Job drawing, mm, ordinate dimensions from the low corner. One solid piece. A direction names the side the tool comes from. Give positions to 0.01 mm unless a question says otherwise; leave off trailing zeros. Loops run counter-clockwise (first coordinate to the right, second up) from the corner with the lowest first, then second, coordinate; pieces in that order, holes last. Notation, with made-up numbers: M -29,39.25 L -3,39.25 A32 ccw -3,76.25 Z; hole C 64,17.25 d11. An arc over 180 degrees is marked long. Put each result on its own line as item: value.
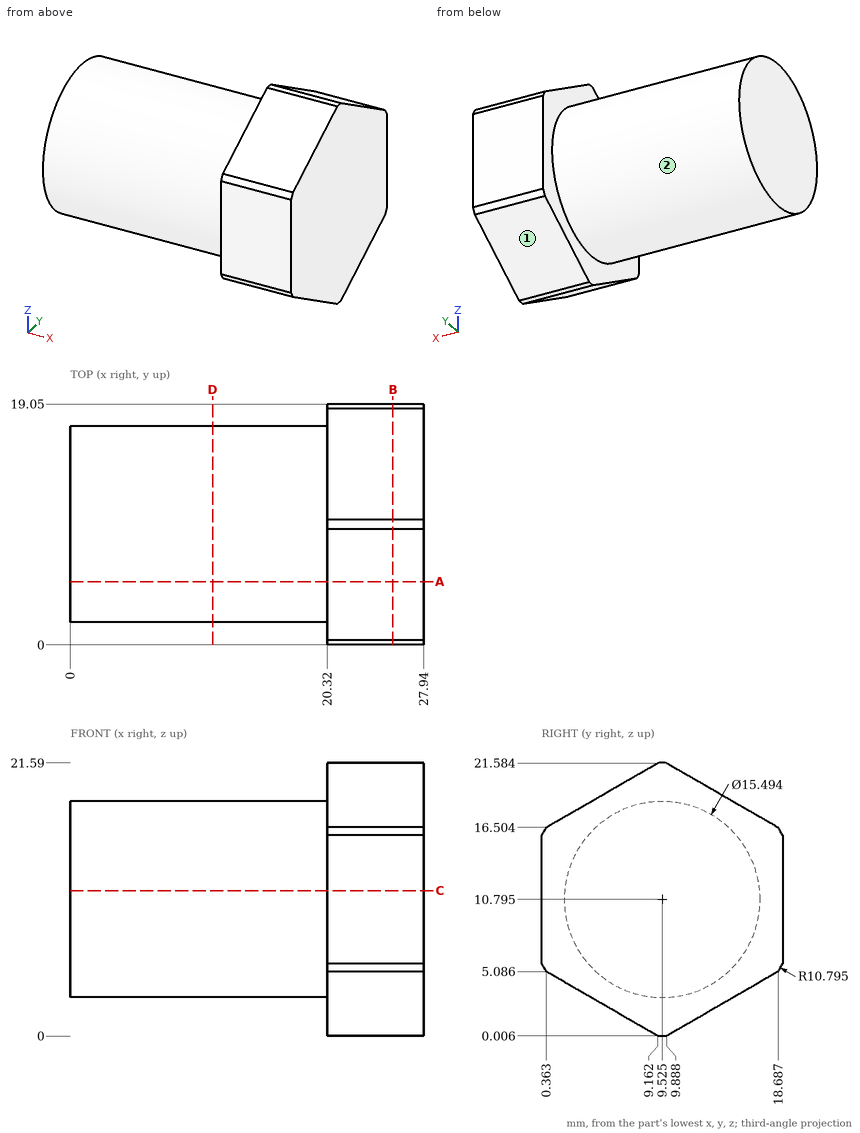
Q1. Slice it at A-A (y = 5). List the corners of the cut face in (x, z).
Here are the results:
outline: M 0,4.51 L 20.32,4.51 L 20.32,2.41 L 27.94,2.41 L 27.94,19.18 L 20.32,19.18 L 20.32,17.08 L 0,17.08 Z
Q2. Drop flat-ended pins along their axis: pin 1 Ø3 at (x, y) = (9, 16) entering from -Z; pin 2 Ø4 at (x, y) = (19.5, 17) entering from -Z; pin 3 Ø6 at (x, z) = (9.5, 5) entering from +Y. Give the stop position or say it passes through.
Here are the results:
pin 1: z = 4.86
pin 2: z = 3.06
pin 3: y = 16.75
Q3. Slice it at D-D (x = 11.25). List the corners of the cut face in (y, z) (3 decimals).
Here are the results:
outline: C 9.525,10.795 d15.494
Q4. Probe line 1 (X direction, y = 2, z = 7.5); line 2 (Z direction, x = 19.75, y = 9.75); line 3 (Z direction, x = 25.5, y = 3.5) (3 decimals). List the from-to ranges inside material, lowest first. Write a range as from..to.
Here are the results:
line 1: 20.32..27.94
line 2: 3.05..18.54
line 3: 3.275..18.315
Q5. Slice it at B-B (x = 25.5). List the corners of the cut face in (y, z) (3 decimals), and give its area (3 significant figures).
Here are the results:
outline: M 0,5.715 A10.795 ccw 0.363,5.086 L 9.162,0.006 A10.795 ccw 9.888,0.006 L 18.687,5.086 A10.795 ccw 19.05,5.715 L 19.05,15.875 A10.795 ccw 18.687,16.504 L 9.888,21.584 A10.795 ccw 9.162,21.584 L 0.363,16.504 A10.795 ccw 0,15.875 Z
area: 314 mm²
Q6. Tool access for the marked faces 1 and 2: list every direction of +Z, -Z, +X, -X, +Y, -Y with a clear straight run to the whole face (end or side of a thin tool).
Here are the results:
face 1: -Z, +X, -X, +Y
face 2: -X
Q7. Slice it at C-C (z = 11.5). List the corners of the cut face in (x, y), and give its area (3 significant figures).
Here are the results:
outline: M 0,1.81 L 20.32,1.81 L 20.32,0 L 27.94,0 L 27.94,19.05 L 20.32,19.05 L 20.32,17.24 L 0,17.24 Z
area: 459 mm²
